Design review of the part built by this model. Coordinates are the model's own, in mm. Round coordinates to 2 decimals unless told otherwise and drop trailing zeros. Order: outer loops, then holes, each group sorted by start corner. A loop starts at its lowest first (then second) coordinate and runs counter-clockwise, first axis right, second up. Notation, with made-up numbers: M 53.5,-25 L 85.5,-25 A28 ccw 85.5,0 Z; hole C -36,41.5 d10. An arc over 180 degrees is marked long. Write item = value, one per line. Start each with the question number.
```python
from build123d import *

# Parameters (mm, degrees)
SKETCH1_R           = 1.75
BOSS_EXTRUDE1_DEPTH = 5
FILLET1_R           = 2


with BuildPart() as part:
    # Sketch1 → Boss-Extrude1 (new body)
    with BuildSketch(Plane.XY):
        with BuildLine():
            Line((-25.5, 3.5), (25.5, 3.5))
            ThreePointArc((25.5, 3.5), (26.914213562, 2.914213562), (27.5, 1.5))
            Line((27.5, 1.5), (27.5, -1.5))
            ThreePointArc((27.5, -1.5), (26.914213562, -2.914213562), (25.5, -3.5))
            Line((25.5, -3.5), (-25.5, -3.5))
            ThreePointArc((-25.5, -3.5), (-26.914213562, -2.914213562), (-27.5, -1.5))
            Line((-27.5, -1.5), (-27.5, 1.5))
            ThreePointArc((-27.5, 1.5), (-26.914213562, 2.914213562), (-25.5, 3.5))
        make_face()
        with Locations((-23.5, 0)):
            Circle(SKETCH1_R, mode=Mode.SUBTRACT)
        with Locations((23.5, 0)):
            Circle(SKETCH1_R, mode=Mode.SUBTRACT)
    extrude(amount=BOSS_EXTRUDE1_DEPTH)

    # Fillet1
    # the kernel refuses this fillet: 2 mm, written as the material it takes off along each edge
    with BuildSketch(Plane(origin=(-25.5, 1.5, 5), x_dir=(-1, 0, 0), z_dir=(0, -1, 0))) as fillet1_piece_1:
        with BuildLine():
            CenterArc((2 - FILLET1_R, FILLET1_R), FILLET1_R, 270, 90)
            Line((2 - FILLET1_R, 0), (2, 0))
            Line((2, 0), (2, FILLET1_R))
        make_face()
    revolve(axis=Axis((-25.5, 1.5, 5), (0, 0, -1)), revolution_arc=90, mode=Mode.SUBTRACT)
    with BuildSketch(Plane(origin=(-27.5, -1.5, 5), x_dir=(0, 0, -1), z_dir=(0, 1, 0)), Plane(origin=(27.5, 1.5, 5), x_dir=(0, 0, -1), z_dir=(0, -1, 0))) as fillet1_piece_2:
        with BuildLine():
            CenterArc((FILLET1_R, -FILLET1_R), FILLET1_R, 90, 90)
            Line((0, -FILLET1_R), (0, 0))
            Line((0, 0), (FILLET1_R, 0))
        make_face()
    extrude(amount=3, mode=Mode.SUBTRACT)
    with BuildSketch(Plane(origin=(-25.5, -1.5, 5), x_dir=(0, -1, 0), z_dir=(1, 0, 0))) as fillet1_piece_3:
        with BuildLine():
            CenterArc((2 - FILLET1_R, FILLET1_R), FILLET1_R, 270, 90)
            Line((2 - FILLET1_R, 0), (2, 0))
            Line((2, 0), (2, FILLET1_R))
        make_face()
    revolve(axis=Axis((-25.5, -1.5, 5), (0, 0, -1)), revolution_arc=90, mode=Mode.SUBTRACT)
    with BuildSketch(Plane(origin=(25.5, -3.5, 5), x_dir=(0, 0, -1), z_dir=(-1, 0, 0)), Plane(origin=(-25.5, 3.5, 5), x_dir=(0, 0, -1), z_dir=(1, 0, 0))) as fillet1_piece_4:
        with BuildLine():
            CenterArc((FILLET1_R, -FILLET1_R), FILLET1_R, 90, 90)
            Line((0, -FILLET1_R), (0, 0))
            Line((0, 0), (FILLET1_R, 0))
        make_face()
    extrude(amount=51, mode=Mode.SUBTRACT)
    with BuildSketch(Plane(origin=(25.5, -1.5, 5), x_dir=(1, 0, 0), z_dir=(0, 1, 0))) as fillet1_piece_5:
        with BuildLine():
            CenterArc((2 - FILLET1_R, FILLET1_R), FILLET1_R, 270, 90)
            Line((2 - FILLET1_R, 0), (2, 0))
            Line((2, 0), (2, FILLET1_R))
        make_face()
    revolve(axis=Axis((25.5, -1.5, 5), (0, 0, -1)), revolution_arc=90, mode=Mode.SUBTRACT)
    with BuildSketch(Plane(origin=(25.5, 1.5, 5), x_dir=(0, 1, 0), z_dir=(-1, 0, 0))) as fillet1_piece_6:
        with BuildLine():
            CenterArc((2 - FILLET1_R, FILLET1_R), FILLET1_R, 270, 90)
            Line((2 - FILLET1_R, 0), (2, 0))
            Line((2, 0), (2, FILLET1_R))
        make_face()
    revolve(axis=Axis((25.5, 1.5, 5), (0, 0, -1)), revolution_arc=90, mode=Mode.SUBTRACT)


solid = part.part
```
(1) Consider section B-B, the plane y = 0. Write out the cut boundary in (x, z), then the cut area to 3 significant figures.
(2) For line 1 along X through (y, z) = (0, 1.35); line 2 along X through (y, z) = (-1.25, 1.4); line 3 along Y through (x, z) = (-23.5, 2.45), list the stretches that pass through material, from the lowest coordinate up. Write a range as [from, to].
(3) Consider section A-A, the plane z = 1.15. Write out the cut boundary in (x, y).
(4) Consider section C-C, the plane x = -23.5. Write out the cut boundary in (y, z), then the cut area to 3 significant figures.
(5) Draft analysis for pull direction X (two halves, no side actions). For faces 1 (the face through (-26.93, -0.02, 4.4)), 2 (the face through (-25.25, 0.08, 2.46)), 3 (the face through (26.93, 0.02, 4.4)), state which applies: pulls with the +X half, pulls with the -X half, needs draft (parallel to the pull), parting line crosses it, or undercut.
(6) Insertion check: pin 1 (1 mm diameter, centred on x = 4, z = 4.5, fed in from +Y); pin 2 (3 mm diameter, centred on x = 23.5, y = 0, fed in from +Z). Each pin has a flat end and moves straight along its axis. Give the tip position at first contact, or say it passes through.
(7) Consider section D-D, the plane y = -3. Write out the cut boundary in (x, z), then the cut area to 3 significant figures.
Completed:
q1.outline = M -27.5,0 L -25.25,0 L -25.25,5 L -25.5,5 A2 ccw -27.5,3 Z; M -21.75,0 L 21.75,0 L 21.75,5 L -21.75,5 Z; M 25.25,0 L 27.5,0 L 27.5,3 A2 ccw 25.5,5 L 25.25,5 Z
q1.area = 238 mm2
q2.line_1 = [-27.5, -25.25], [-21.75, 21.75], [25.25, 27.5]
q2.line_2 = [-27.5, -24.72], [-22.28, 22.28], [24.72, 27.5]
q2.line_3 = [-3.5, -1.75], [1.75, 3.5]
q3.outline = M -27.5,-1.5 A2 ccw -25.5,-3.5 L 25.5,-3.5 A2 ccw 27.5,-1.5 L 27.5,1.5 A2 ccw 25.5,3.5 L -25.5,3.5 A2 ccw -27.5,1.5 Z; hole C -23.5,0 d3.5; hole C 23.5,0 d3.5
q4.outline = M -3.5,0 L -1.75,0 L -1.75,4.98 A2 ccw -3.5,3 Z; M 1.75,0 L 3.5,0 L 3.5,3 A2 ccw 1.75,4.98 Z
q4.area = 15.8 mm2
q5.face_1 = pulls with the -X half
q5.face_2 = undercut
q5.face_3 = pulls with the +X half
q6.pin_1 = 3.23
q6.pin_2 = through
q7.outline = M -26.82,0 L 26.82,0 L 26.82,3 A1.32 ccw 25.5,4.32 L -25.5,4.32 A1.32 ccw -26.82,3 Z
q7.area = 231 mm2
